from build123d import *

# Parameters (mm, degrees)
AUFSATZ_LINEAR_AUSTRAGEN1_DEPTH      = 10
SKIZZE3_W                            = 136
SKIZZE3_H                            = 8.65
AUFSATZ_LINEAR_AUSTRAGEN2_DEPTH      = 10
SCHNITT_LINEAR_AUSTRAGEN1_DEPTH      = 10
SCHNITT_LINEAR_AUSTRAGEN1_DEPTH_BACK = 10
BOHRUNG1_D                           = 6
BOHRUNG2_D                           = 4.134
BOHRUNG2_DEPTH                       = 10
BOHRUNG2_CSINK_D                     = 5
BOHRUNG2_CSINK_ANGLE                 = 90
BOHRUNG3_D                           = 4.134
BOHRUNG3_DEPTH                       = 11
BOHRUNG3_CSINK_D                     = 5
BOHRUNG3_CSINK_ANGLE                 = 90
BOHRUNG3_TIP                         = 1.193383006


with BuildPart() as part:
    # Skizze1 → Rotation1 (revolve)
    with BuildSketch(Plane.XY, mode=Mode.PRIVATE) as rotation1_sk:
        with BuildLine():
            Line((0, 0), (0, 6.8))
            Line((0, 6.8), (0.2, 7))
            Line((0.2, 7), (1, 7))
            Line((1, 7), (2, 8))
            Line((2, 8), (11.95, 8))
            Line((11.95, 8), (12.865685425, 7.084314575))
            ThreePointArc((12.865685425, 7.084314575), (13.125224104, 6.910896374), (13.43137085, 6.85))
            Line((13.43137085, 6.85), (14.2, 6.85))
            ThreePointArc((14.2, 6.85), (14.765685425, 7.084314575), (15, 7.65))
            Line((15, 7.65), (15, 8))
            Line((15, 8), (17, 8))
            Line((17, 8), (17, 0))
            Line((17, 0), (0, 0))
        make_face()
    revolve(rotation1_sk.sketch.rotate(Axis((17, 0, 0), (-1, 0, 0)), 270), axis=Axis((17, 0, 0), (-1, 0, 0)))

    # Skizze2 → Aufsatz-Linear austragen1 (add)
    with BuildSketch(Plane(origin=(17, 0, 0), x_dir=(0, 0, -1), z_dir=(1, 0, 0))):
        with BuildLine():
            Line((4.75, 8.977054082), (4.75, 9.6))
            ThreePointArc((4.75, 9.6), (4.632842712, 9.882842712), (4.35, 10))
            Line((4.35, 10), (-4.35, 10))
            ThreePointArc((-4.35, 10), (-4.632842712, 9.882842712), (-4.75, 9.6))
            Line((-4.75, 9.6), (-4.75, 8.977054082))
            ThreePointArc((-4.75, 8.977054082), (-4.791034545, 8.825604773), (-4.902912621, 8.715586488))
            ThreePointArc((-4.902912621, 8.715586488), (0, -10), (4.902912621, 8.715586488))
            ThreePointArc((4.902912621, 8.715586488), (4.791034545, 8.825604773), (4.75, 8.977054082))
        make_face()
    extrude(amount=AUFSATZ_LINEAR_AUSTRAGEN1_DEPTH)

    # Skizze3 → Rotation2 (revolve)
    with BuildSketch(Plane.XY, mode=Mode.PRIVATE) as rotation2_sk:
        with Locations((95, 4.325)):
            Rectangle(SKIZZE3_W, SKIZZE3_H)
    revolve(rotation2_sk.sketch.rotate(Axis((163, 0, 0), (-1, 0, 0)), 270), axis=Axis((163, 0, 0), (-1, 0, 0)))

    # Skizze4 → Aufsatz-Linear austragen2 (add)
    with BuildSketch(Plane(origin=(163, 0, 0), x_dir=(0, 0, -1), z_dir=(1, 0, 0))):
        with BuildLine():
            Line((4.75, 8.977054082), (4.75, 9.6))
            ThreePointArc((4.75, 9.6), (4.632842712, 9.882842712), (4.35, 10))
            Line((4.35, 10), (-4.35, 10))
            ThreePointArc((-4.35, 10), (-4.632842712, 9.882842712), (-4.75, 9.6))
            Line((-4.75, 9.6), (-4.75, 8.977054082))
            ThreePointArc((-4.75, 8.977054082), (-4.791034545, 8.825604773), (-4.902912621, 8.715586488))
            ThreePointArc((-4.902912621, 8.715586488), (0, -10), (4.902912621, 8.715586488))
            ThreePointArc((4.902912621, 8.715586488), (4.791034545, 8.825604773), (4.75, 8.977054082))
        make_face()
    extrude(amount=AUFSATZ_LINEAR_AUSTRAGEN2_DEPTH)

    # Skizze5 → Rotation3 (revolve)
    with BuildSketch(Plane.XY, mode=Mode.PRIVATE) as rotation3_sk:
        with BuildLine():
            Line((173, 0), (173, 8))
            Line((173, 8), (175, 8))
            Line((175, 8), (175, 7.65))
            ThreePointArc((175, 7.65), (175.234314575, 7.084314575), (175.8, 6.85))
            Line((175.8, 6.85), (176.56862915, 6.85))
            ThreePointArc((176.56862915, 6.85), (176.874775896, 6.910896374), (177.134314575, 7.084314575))
            Line((177.134314575, 7.084314575), (178.05, 8))
            Line((178.05, 8), (188, 8))
            Line((188, 8), (189, 7))
            Line((189, 7), (189.8, 7))
            Line((189.8, 7), (190, 6.8))
            Line((190, 6.8), (190, 0))
            Line((190, 0), (173, 0))
        make_face()
    revolve(rotation3_sk.sketch.rotate(Axis((190, 0, 0), (-1, 0, 0)), 270), axis=Axis((190, 0, 0), (-1, 0, 0)))

    # Skizze6 → Schnitt-Linear austragen1 (cut, two sides: drawn at the far end of the back side and taken through both)
    with BuildSketch(Plane(origin=(0, 0, 0), x_dir=(1, 0, 0), z_dir=(0, 1, 0)).offset(-SCHNITT_LINEAR_AUSTRAGEN1_DEPTH_BACK)):
        Polygon((168, 18), (168, 6), (190, 6), (190, -6), (168, -6), (168, -18), (202, -18), (202, 18), align=None)
    extrude(amount=SCHNITT_LINEAR_AUSTRAGEN1_DEPTH + SCHNITT_LINEAR_AUSTRAGEN1_DEPTH_BACK, mode=Mode.SUBTRACT)

    # Bohrung1 (through all)
    with Locations(Plane(origin=(0, 0, -6), x_dir=(-1, 0, 0), z_dir=(0, 0, -1))):
        with Locations((-177, 0)):
            Hole(BOHRUNG1_D / 2)

    # Bohrung2
    with Locations(Plane(origin=(0, 10, 0), x_dir=(1, 0, 0), z_dir=(0, 1, 0))):
        with Locations((23, 0)):
            CounterSinkHole(BOHRUNG2_D / 2, BOHRUNG2_CSINK_D / 2, depth=BOHRUNG2_DEPTH, counter_sink_angle=BOHRUNG2_CSINK_ANGLE)

    # Bohrung3
    with Locations(Plane(origin=(0, 10, 0), x_dir=(1, 0, 0), z_dir=(0, 1, 0))):
        with Locations((167, 0)):
            CounterSinkHole(BOHRUNG3_D / 2, BOHRUNG3_CSINK_D / 2, depth=BOHRUNG3_DEPTH, counter_sink_angle=BOHRUNG3_CSINK_ANGLE)
            with Locations((0, 0, -(BOHRUNG3_DEPTH + BOHRUNG3_TIP / 2))):  # 120° drill point
                Cone(0, BOHRUNG3_D / 2, BOHRUNG3_TIP, mode=Mode.SUBTRACT)

    # Skizze13 → Schnitt-Rotation1 (revolve, cut)
    with BuildSketch(Plane.XY, mode=Mode.PRIVATE) as schnitt_rotation1_sk:
        Polygon((-5, 0), (-5, 3), (41.2, 3), (41.2, 8), (145.2, 8), (145.2, 0), align=None)
    revolve(schnitt_rotation1_sk.sketch.rotate(Axis((145.2, 0, 0), (-1, 0, 0)), 270), axis=Axis((145.2, 0, 0), (-1, 0, 0)), mode=Mode.SUBTRACT)


solid = part.part
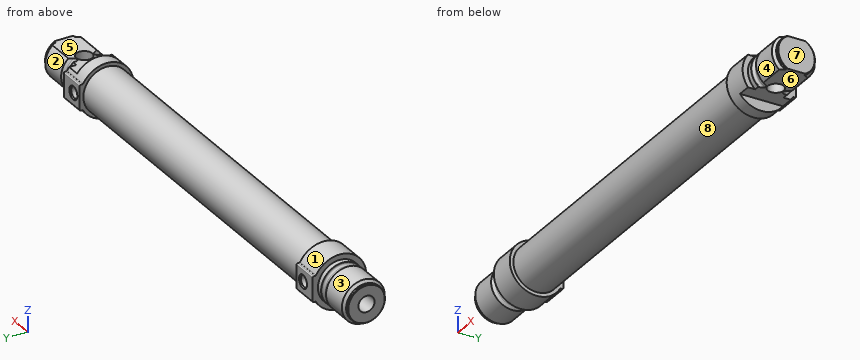
Verification items for the finished model (mm, model axes). Face numbers are marked on the shaded views. A direction names the side the tool comes from. Round coordinates to 2 decimals unless told otherwise and drop trailing zeros. Order: outer loops, then holes, each group sorted by start corner. A loop starts at its lowest first (then second) coordinate and runs counter-clockwise, first axis right, second up.
1. Section check A-A on x = 23. Record the cut outline in (y, z).
Final values:
outline: (2.17, -2.07) arc R3 cw (long way) to (2.17, 2.07) - (9.57, 2.07) - (10, 2.5) - (10, 4.35) arc R0.4 ccw to (9.6, 4.75) - (8.98, 4.75) arc R0.3 cw to (8.72, 4.9) arc R10 ccw (long way) to (8.72, -4.9) arc R0.3 cw to (8.98, -4.75) - (9.6, -4.75) arc R0.4 ccw to (10, -4.35) - (10, -2.5) - (9.57, -2.07) - close
2. Thickness scan on L1, parallel to X at y = -3.5, z = 2.5; L2, parallel to X at y = -0.5, z = 3.75; L3, parallel to X at y = 8, z = 4. Record the ranges inside material, lowest first.
Final values:
L1: x = 0 to 41.2, 145.2 to 190
L2: x = 0 to 41.2, 145.2 to 174.04, 179.96 to 190
L3: x = 17 to 27, 163 to 173
3. Go/stop test with flat-tipped pins: P1, Ø3, axis at y = 4, z = 8, coming from the +X side; P2, Ø1.5, axis at x = 63.5, z = -6.5, coming from the -Y side; P3, Ø8, axis at x = 176, y = -1.5, coming from the -Z side. Record where each tip stops, or that it passes through.
Final values:
P1: stops at x = 168
P2: stops at y = -6.46
P3: stops at z = -6
4. Access from +Z, -Z, +X, -X, +Y, -Y to the whole of each face (thin tool, end or side, straight path). Record for the marked faces 1, 2, 3, 4 and 5.
Final values:
face 1: +X, -X
face 2: +X, +Y
face 3: -X
face 4: +X, -Y
face 5: +Z, +X, +Y, -Y
5. Release check for a two-part mould opening along X. For the marked faces 6, 7 and 8 record: +X half, -X half, draft (parallel to the pull), parting line (faces both ways), or undercut.
Final values:
face 6: draft
face 7: +X half
face 8: undercut
6. Section check B-B on x = 104. Record the cut outline in (y, z), then the cut area to 3 significant figures.
Final values:
outline: circle Ø17.3 at (0, 0); hole circle Ø16 at (0, 0)
area: 34.0 mm2
